Could you check a few things on this model? Use its own coordinates, in mm. A direction names the side the tool comes from. Round coordinates to 2 decimals unless told otherwise and drop trailing zeros. Loops run counter-clockwise (first coordinate to the right, second up) from the corner with the lowest first, then second, coordinate; pieces in that order, holes last. Notation, with made-up numbers: (23.25, 76.25) - (57.25, 76.25) arc R33 ccw to (57.25, 115.25) - close; hole circle Ø1 at (-1, 57). An arc over 180 degrees is marked (long way). Answer as CSV lines item,"result". Start each with the question number.
1) I'm going to push flat-ended pins straight in: pin 1 Ø4 at (y, z) = (6.5, 32.5) entering from +X; pin 2 Ø1.2 at (x, z) = (-1.5, 38.5) entering from +Y; pin 3 Ø4.5 at (x, z) = (-12.5, 18.5) entering from +Y; pin 4 Ø1.2 at (x, y) = (-18.5, 38) entering from +Z. Where does each tip first touch, or does it pass through?
2) Which directions (+Z, -Z, +X, -X, +Y, -Y) give clear straight access to the entire face, cutting with the end or side of a thin tool? Please do faces 1 (the face through (-1, 39, 6.5)), 2 (the face through (-10, 0, 20)), 3 (the face through (-10, 22, 4)).
3) We'd pull the mould along Z, two halves only. Please class faces 4 (the face through (-11.48, 2.03, 32.32)), 5 (the face through (0, 15, 16)), 6 (the face through (-10, 20, 0)): pulls with the +Z half, pulls with the -Z half, needs draft (parallel to the pull), parting line crosses it, or undercut.
4) Suppose I cut it at A-A, the plane y = 10. Write out the boundary of the cut face in (x, z), then the cut area to 4 significant figures.
5) Please list where these lines run through material, in increasing order: line 1 along Z through (x, y) = (-10, 2.5); line 2 along X through (y, z) = (6, 14.5).
6) Suppose I cut it at B-B, the plane x = -10. Write out the boundary of the cut face in (y, z), then the cut area to 3 significant figures.
7) Suppose I cut it at C-C, the plane z = 30. Write out the boundary of the cut face in (x, y), then the cut area to 4 significant figures.
8) Suppose I cut it at D-D, the plane z = 16. Write out the boundary of the cut face in (x, y), then the cut area to 4 significant figures.
```python
from build123d import *

# Parameters (mm, degrees)
F0_W     = 20
F0_H     = 40
F1_DEPTH = 4
F2_W     = 20
F2_H     = 40
F3_DEPTH = 4
F7_DEPTH = 2.5
F8_DEPTH = 2.5
F9_D     = 5.5
F11_D    = 5.5


with BuildPart() as f1:
    # F0 (on Top) → F1 (new body)
    with BuildSketch(Plane.XY):
        with Locations((-10, 20)):
            Rectangle(F0_W, F0_H)
    extrude(amount=F1_DEPTH)

    # F2 (on Front) → F3 (join)
    with BuildSketch(Plane.XZ):
        with Locations((-10, 20)):
            Rectangle(F2_W, F2_H)
    extrude(amount=-F3_DEPTH)

    # F6 (on face) → F7 (join)
    with BuildSketch(Plane(origin=(-20, 0, 0), x_dir=(0, -1, 0), z_dir=(-1, 0, 0))):
        Polygon((-4, 4), (-4, 40), (-6.5, 40), (-6.5, 37), (-37, 6.5), (-40, 6.5), (-40, 4), align=None)
    extrude(amount=-F7_DEPTH)

    # F5 (on face) → F8 (join)
    with BuildSketch(Plane.YZ):
        Polygon((4, 4), (40, 4), (40, 6.5), (37, 6.5), (6.5, 37), (6.5, 40), (4, 40), align=None)
    extrude(amount=-F8_DEPTH)

    # F9 (through all)
    with Locations(Plane.XZ):
        with Locations((-10, 30), (-10, 10)):
            Hole(F9_D / 2)

    # F11 (through all)
    with Locations(Plane(origin=(0, 0, 0), x_dir=(1, 0, 0), z_dir=(0, 0, -1))):
        with Locations((-10, -30), (-10, -10)):
            Hole(F11_D / 2)


solid = f1.part
```
Filled sheet:
1,pin 1,"x = 0"
1,pin 2,"y = 6.5"
1,pin 3,"y = 4"
1,pin 4,"z = 6.5"
2,face 1,"+Z, +X, -X, +Y"
2,face 2,"+Z, -Z, +X, -X, -Y"
2,face 3,"+Z, +Y"
3,face 4,"undercut"
3,face 5,"needs draft"
3,face 6,"pulls with the -Z half"
4,outline,"(-20, 0) - (-12.75, 0) - (-12.75, 4) - (-17.5, 4) - (-17.5, 33.5) - (-20, 33.5) - close; (-7.25, 0) - (0, 0) - (0, 33.5) - (-2.5, 33.5) - (-2.5, 4) - (-7.25, 4) - close"
4,area,"205.5 mm²"
5,line 1,"0 to 7.25, 12.75 to 27.25, 32.75 to 40"
5,line 2,"-20 to -17.5, -2.5 to 0"
6,outline,"(0, 0) - (7.25, 0) - (7.25, 4) - (4, 4) - (4, 7.25) - (0, 7.25) - close; (0, 12.75) - (4, 12.75) - (4, 27.25) - (0, 27.25) - close; (0, 32.75) - (4, 32.75) - (4, 40) - (0, 40) - close; (12.75, 0) - (27.25, 0) - (27.25, 4) - (12.75, 4) - close; (32.75, 0) - (40, 0) - (40, 4) - (32.75, 4) - close"
6,area,"216 mm²"
7,outline,"(-20, 0) - (-12.75, 0) - (-12.75, 4) - (-17.5, 4) - (-17.5, 13.5) - (-20, 13.5) - close; (-7.25, 0) - (0, 0) - (0, 13.5) - (-2.5, 13.5) - (-2.5, 4) - (-7.25, 4) - close"
7,area,"105.5 mm²"
8,outline,"(-20, 0) - (0, 0) - (0, 27.5) - (-2.5, 27.5) - (-2.5, 4) - (-17.5, 4) - (-17.5, 27.5) - (-20, 27.5) - close"
8,area,"197.5 mm²"
